from build123d import *

# Parameters (mm, degrees)
CROQUIS1_W              = 40
CROQUIS1_H              = 40
SALIENTE_EXTRUIR1_DEPTH = 2
CROQUIS2_W              = 40
CROQUIS2_H              = 40
CROQUIS2_W_2            = 29
CROQUIS2_H_2            = 29
SALIENTE_EXTRUIR2_DEPTH = 15
CROQUIS3_W              = 59
CROQUIS3_H              = 59
CROQUIS3_W_2            = 29
CROQUIS3_H_2            = 29
SALIENTE_EXTRUIR3_DEPTH = 5
CORTAR_EXTRUIR1_DEPTH   = 20
CROQUIS5_R              = 1.6
CORTAR_EXTRUIR2_DEPTH   = 5
CROQUIS6_W              = 30
CROQUIS6_H              = 30
CORTAR_EXTRUIR3_DEPTH   = 1
CROQUIS7_W              = 3
CROQUIS7_H              = 3
CORTAR_EXTRUIR4_DEPTH   = 5


with BuildPart() as part:
    # Croquis1 → Saliente-Extruir1 (new body)
    with BuildSketch(Plane(origin=(0, 0, 0), x_dir=(1, 0, 0), z_dir=(0, 1, 0))):
        with Locations((20, 20)):
            Rectangle(CROQUIS1_W, CROQUIS1_H)
    extrude(amount=SALIENTE_EXTRUIR1_DEPTH)

    # Croquis2 → Saliente-Extruir2 (add)
    with BuildSketch(Plane(origin=(0, 2, 0), x_dir=(1, 0, 0), z_dir=(0, 1, 0))):
        with Locations((20, 20)):
            Rectangle(CROQUIS2_W, CROQUIS2_H)
        with Locations((20, 20)):
            Rectangle(CROQUIS2_W_2, CROQUIS2_H_2, mode=Mode.SUBTRACT)
    extrude(amount=SALIENTE_EXTRUIR2_DEPTH)

    # Croquis3 → Saliente-Extruir3 (add)
    with BuildSketch(Plane(origin=(0, 17, 0), x_dir=(1, 0, 0), z_dir=(0, 1, 0))):
        with Locations((20, 20)):
            Rectangle(CROQUIS3_W, CROQUIS3_H)
        with Locations((20, 20)):
            Rectangle(CROQUIS3_W_2, CROQUIS3_H_2, mode=Mode.SUBTRACT)
    extrude(amount=SALIENTE_EXTRUIR3_DEPTH)

    # Croquis4 → Cortar-Extruir1 (cut)
    with BuildSketch(Plane(origin=(0, 22, 0), x_dir=(1, 0, 0), z_dir=(0, 1, 0))):
        Polygon((19.4, 5.5), (19.4, 3.5), (20.6, 3.5), (20.6, 5.5), (34.5, 5.5), (34.5, 19.4), (36.5, 19.4), (36.5, 20.6), (34.5, 20.6), (34.5, 34.5), (20.6, 34.5), (20.6, 36.5), (19.4, 36.5), (19.4, 34.5), (5.5, 34.5), (5.5, 20.6), (3.5, 20.6), (3.5, 19.4), (5.5, 19.4), (5.5, 5.5), align=None)
    extrude(amount=-CORTAR_EXTRUIR1_DEPTH, mode=Mode.SUBTRACT)

    # Croquis5 → Cortar-Extruir2 (cut)
    with BuildSketch(Plane.XZ.offset(-17)):
        with Locations(Location((-4.75, 4.75, 0), (0, 0, 270))):
            Circle(CROQUIS5_R)
        with Locations(Location((44.75, 4.75, 0), (0, 0, 270))):
            Circle(CROQUIS5_R)
        with Locations(Location((44.75, -44.75, 0), (0, 0, 270))):
            Circle(CROQUIS5_R)
        with Locations(Location((-4.75, -44.75, 0), (0, 0, 270))):
            Circle(CROQUIS5_R)
    extrude(amount=-CORTAR_EXTRUIR2_DEPTH, mode=Mode.SUBTRACT)

    # Croquis6 → Cortar-Extruir3 (cut)
    with BuildSketch(Plane(origin=(0, 22, 0), x_dir=(1, 0, 0), z_dir=(0, 1, 0))):
        with Locations((20, 20)):
            Rectangle(CROQUIS6_W, CROQUIS6_H)
    extrude(amount=-CORTAR_EXTRUIR3_DEPTH, mode=Mode.SUBTRACT)

    # Croquis7 → Cortar-Extruir4 (cut)
    with BuildSketch(Plane(origin=(0, 2, 0), x_dir=(1, 0, 0), z_dir=(0, 1, 0))):
        with Locations((33, 7)):
            Rectangle(CROQUIS7_W, CROQUIS7_H)
    extrude(amount=-CORTAR_EXTRUIR4_DEPTH, mode=Mode.SUBTRACT)


solid = part.part
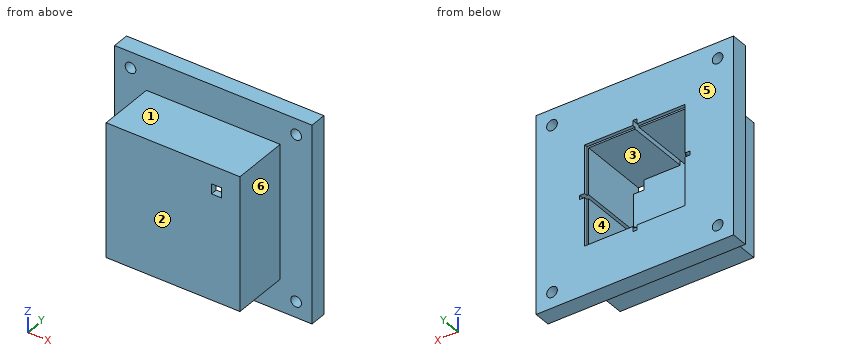
Build history of the part. All positions in model axes, mm. Face numbers are marked on the shaded views. A direction names the side the tool comes from. Round coordinates to 2 decimals unless told otherwise and drop trailing zeros. Loops run counter-clockwise (first coordinate to the right, second up) from the corner with the lowest first, then second, coordinate; pieces in that order, holes last. Notation, with made-up numbers: (-30.75, 53) -> (15.25, 53) arc R19 ccw to (15.25, 75) -> close; hole circle Ø4 at (59.5, 59). An arc over 180 degrees is marked (long way). Use CSV: the item, a comma, the result in double quotes. Start each with the question number.
Q1. Mould opens along Z. For the marked faces 1, 2 and 3 say: +Z half, -Z half, draft (parallel to the pull), parting line (faces both ways), or undercut.
Q2. Saw through at B-B on y = 20. Give the cut face in (x, z).
Q3. Which spindle directions (+Z, -Z, +X, -X, +Y, -Y) get a long thin tool onto all of the face, cutting with end or side? Do the marked faces 4, 5 and 6. Say none if no direction does.
Q4. Saw through at A-A on z = -44.75. Give the cut face in (x, y).
Q5. Saw through at D-D on z = -24. Give the cut face in (x, y), and give its area (3 significant figures).
Q6. Flat gauge pins, fed straight in: pin 1 Ø8 at (y, z) = (5, -7) entering from +X; pin 2 Ø8 at (y, z) = (12.5, -40) entering from -X; pin 3 Ø5 at (x, y) = (14, 6.5) entering from -Z; pin 4 Ø3 at (x, z) = (44.75, -44.75) entering from +Y. Where does each tip first touch, or does it go through?
Q7. Drill centre lines: L1, parallel to X at y = 18.2, z = 4.75; L2, parallel to X at y = 9, z = -6.5; L3, parallel to X at y = 20.75, z = -33.5. Where is each one in solid material? Low to high.
Q8. Saw through at C-C on x = -4.75. Give the cut face in (y, z), and give its area (3 significant figures).
Solutions:
1,face 1,"+Z half"
1,face 2,"draft"
1,face 3,"undercut"
2,outline,"(-9.5, -49.5) -> (49.5, -49.5) -> (49.5, 9.5) -> (-9.5, 9.5) -> close; hole circle Ø3.2 at (-4.75, -44.75); hole circle Ø3.2 at (-4.75, 4.75); hole (3.5, -20.6) -> (5.5, -20.6) -> (5.5, -34.5) -> (19.4, -34.5) -> (19.4, -36.5) -> (20.6, -36.5) -> (20.6, -34.5) -> (34.5, -34.5) -> (34.5, -20.6) -> (36.5, -20.6) -> (36.5, -19.4) -> (34.5, -19.4) -> (34.5, -5.5) -> (20.6, -5.5) -> (20.6, -3.5) -> (19.4, -3.5) -> (19.4, -5.5) -> (5.5, -5.5) -> (5.5, -19.4) -> (3.5, -19.4) -> close; hole circle Ø3.2 at (44.75, -44.75); hole circle Ø3.2 at (44.75, 4.75)"
3,face 4,"+Y"
3,face 5,"+Z, -Z, +X, -X, +Y"
3,face 6,"+Z, -Z, +X, -Y"
4,outline,"(-9.5, 17) -> (-6.35, 17) -> (-6.35, 22) -> (-9.5, 22) -> close; (-3.15, 17) -> (43.15, 17) -> (43.15, 22) -> (-3.15, 22) -> close; (46.35, 17) -> (49.5, 17) -> (49.5, 22) -> (46.35, 22) -> close"
5,outline,"(-9.5, 17) -> (0, 17) -> (0, 0) -> (40, 0) -> (40, 17) -> (49.5, 17) -> (49.5, 22) -> (35, 22) -> (35, 21) -> (34.5, 21) -> (34.5, 2) -> (5.5, 2) -> (5.5, 21) -> (5, 21) -> (5, 22) -> (-9.5, 22) -> close"
5,area,"394 mm^2"
6,pin 1,"stops at x = 40"
6,pin 2,"stops at x = 0"
6,pin 3,"stops at z = -40"
6,pin 4,"passes through"
7,L1,"x = -9.5 to -6.35, -3.15 to 43.15, 46.35 to 49.5"
7,L2,"x = 0 to 5.5, 34.5 to 40"
7,L3,"x = -9.5 to 5.5, 34.5 to 49.5"
8,outline,"(17, -49.5) -> (22, -49.5) -> (22, -46.35) -> (17, -46.35) -> close; (17, -43.15) -> (22, -43.15) -> (22, 3.15) -> (17, 3.15) -> close; (17, 6.35) -> (22, 6.35) -> (22, 9.5) -> (17, 9.5) -> close"
8,area,"263 mm^2"
